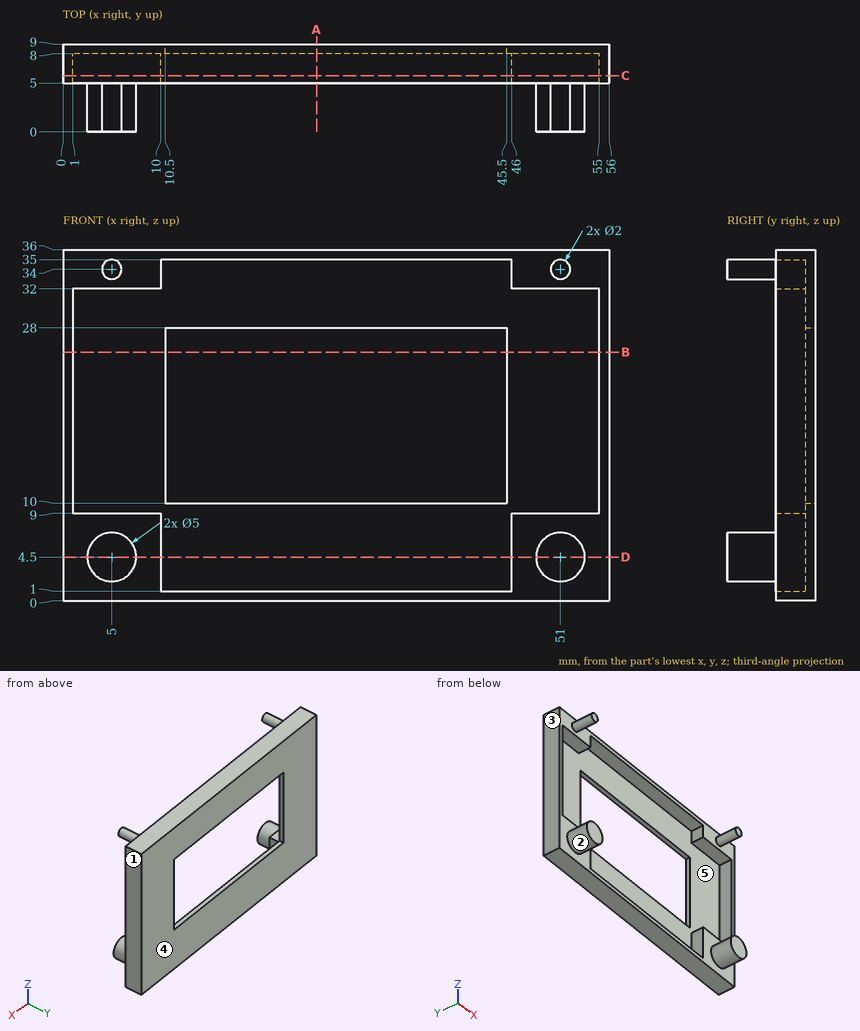
Input: dimensioned drawing with shaded views. Units: mm. Origin: part minimum x, y, z. A direction names the side the tool comes from. Coordinates: 2 decimals unless noted, no trailing zeros. Write each loop counter-clockwise with the first axis right and the second up, starting at its lowest first coordinate (ties: lowest second). Pieces come first, ordered by that corner, then holes. Notation, with made-up numbers: (8.25, 44.25) -> (41.25, 44.25) arc R14 ccw to (41.25, 58.25) -> close; hole circle Ø7 at (44.5, 72.25). An arc over 180 degrees is marked (long way). Return JSON: item names as keys, results as strings. Group by question number.
1) Ray query, line 1 along Z through (x, y) = (15.5, 6.75); line 2 along Z through (x, y) = (9.5, 6.5); line 3 along X through (y, z) = (7, 7.5). Return the intervals inside material, ascending.
2) Section query C-C, the plane y = 5.75. Return loops of the section in (x, z), plus the area to 3 significant figures.
3) Section query B-B, the plane z = 25.5. Return loops of the section in (x, y).
4) Section query D-D, the plane z = 4.5. Return loops of the section in (x, y), plus the area to 3 significant figures.
5) Set-up query: the marked faces 4 and 5. Return all of +Z, -Z, +X, -X, +Y, -Y with unobstructed straight access to the full face (end or side cutting, diameter ignored); none if empty.
6) Section query A-A, the plane x = 26. Return loops of the section in (y, z), plus the area to 3 significant figures.
7) Contact query for a flat-ended pin moving along its axis: P1, Ø1, axis at x = 12.5, z = 30, coming from the -Y side. Output: stop coordinate, or through.
8) Mould query, pull axis X, two halves, no side actions, for the marked faces 1, 2 and 3. Classes: +X half, -X half, draft (parallel to the pull), parting line (faces both ways), or undercut.
From the geometry:
{
 "1": {"line 1": "0 to 1, 35 to 36", "line 2": "0 to 9, 32 to 36", "line 3": "0 to 10, 46 to 56"},
 "2": {"outline": "(0, 0) -> (56, 0) -> (56, 36) -> (0, 36) -> close; hole (1, 9) -> (10, 9) -> (10, 1) -> (46, 1) -> (46, 9) -> (55, 9) -> (55, 32) -> (46, 32) -> (46, 35) -> (10, 35) -> (10, 32) -> (1, 32) -> close", "area": "378 mm²"},
 "3": {"outline": "(0, 5) -> (1, 5) -> (1, 8) -> (10.5, 8) -> (10.5, 9) -> (0, 9) -> close; (45.5, 8) -> (55, 8) -> (55, 5) -> (56, 5) -> (56, 9) -> (45.5, 9) -> close"},
 "4": {"outline": "(0, 5) -> (2.5, 5) -> (2.5, 0) -> (7.5, 0) -> (7.5, 5) -> (10, 5) -> (10, 8) -> (46, 8) -> (46, 5) -> (48.5, 5) -> (48.5, 0) -> (53.5, 0) -> (53.5, 5) -> (56, 5) -> (56, 9) -> (0, 9) -> close", "area": "166 mm²"},
 "5": {"face 4": "+Z, -Z, +X, -X, +Y", "face 5": "-Y"},
 "6": {"outline": "(5, 0) -> (9, 0) -> (9, 10) -> (8, 10) -> (8, 1) -> (5, 1) -> close; (5, 35) -> (8, 35) -> (8, 28) -> (9, 28) -> (9, 36) -> (5, 36) -> close", "area": "24.0 mm²"},
 "7": {"P1": "y = 8"},
 "8": {"face 1": "+X half", "face 2": "undercut", "face 3": "-X half"}
}
